Verification items for this drawing (mm, ordinates from the low corner). A direction names the side the tool comes from. Give positions to 0.01 mm unless a question says otherwise; leave off trailing zeros. Order: outer loops, then holes, each group sorted by start corner. A loop starts at its lowest first (then second) coordinate and runs counter-clockwise, first axis right, second up.
(1) Sectioned sample at C-C on y = 18.25. Record the cut outline in (x, z).
(2) Access from +Z, -Z, +X, -X, +Y, -Y to the whole of each face (thin tool, end or side, straight path). Record for the marked faces 5, 6 and 7.
(3) Sectioned sample at B-B on z = 31.5. Record the cut outline in (x, y).
(4) Mould release check, pull along X, two halves, no side actions. Record for the marked faces 1, 2, 3 and 4: pulls with the +X half, pulls with the -X half, needs draft (parallel to the pull), parting line crosses it, or undercut.
(5) Sectioned sample at A-A on x = 29. Record the cut outline in (y, z), plus the area to 3 significant figures.
(6) Scan lines: L1, parallel to Z at x = 39.5, y = 2.5; L2, parallel to X at y = 8.25, z = 25.5; L3, parallel to X at y = 16.25, z = 22. Record each from-to range of solid material in increasing order.
(7) Sectioned sample at D-D on x = 35. Record the cut outline in (y, z).
(8) Gauge pin test, flat ends, axial feed: pin 1 (6.5 mm diameter, centred on y = 5.5, z = 29.5, fed in from +X); pin 2 (10 mm diameter, centred on x = 39.5, z = 24.5, fed in from -Y). Record the tip position at first contact, or that the pin passes through.
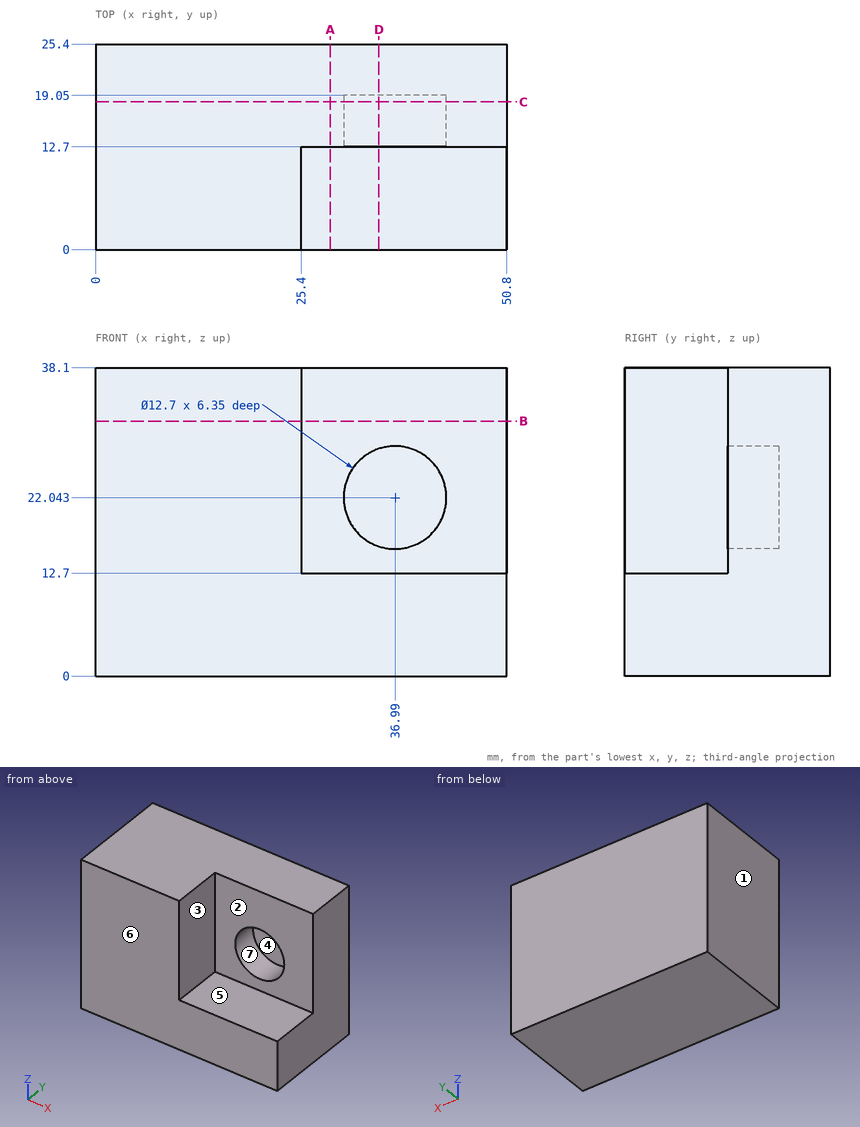
Ans:
1. outline: (0, 0) - (50.8, 0) - (50.8, 38.1) - (0, 38.1) - close; hole circle Ø12.7 at (36.99, 22.04)
2. face 5: +Z, +X, -Y
2. face 6: +Z, -Z, +X, -X, -Y
2. face 7: -Y
3. outline: (0, 0) - (25.4, 0) - (25.4, 12.7) - (50.8, 12.7) - (50.8, 25.4) - (0, 25.4) - close
4. face 1: pulls with the -X half
4. face 2: needs draft
4. face 3: pulls with the +X half
4. face 4: undercut
5. outline: (0, 0) - (25.4, 0) - (25.4, 38.1) - (12.7, 38.1) - (12.7, 12.7) - (0, 12.7) - close
5. area: 645 mm2
6. L1: z = 0 to 12.7
6. L2: x = 0 to 25.4
6. L3: x = 0 to 30.64, 43.34 to 50.8
7. outline: (0, 0) - (25.4, 0) - (25.4, 38.1) - (12.7, 38.1) - (12.7, 28.07) - (19.05, 28.07) - (19.05, 16.01) - (12.7, 16.01) - (12.7, 12.7) - (0, 12.7) - close
8. pin 1: stops at x = 25.4
8. pin 2: stops at y = 12.7
